Build history of the part. All positions in model axes, mm. A direction names the side the tool comes from. Give positions to 0.01 mm unless a question says otherwise; leave off trailing zeros. Order: outer loops, then holes, each group sorted by start corner. A loop starts at its lowest first (then second) coordinate and runs counter-clockwise, first axis right, second up. Notation, with made-up numbers: (31, 80) -> (44, 80) arc R16 ccw to (44, 98) -> close; hole circle Ø2 at (-24, 47). An arc over 180 degrees is marked (long way). Use a Markdown table: item, result. Add a question column.
Autodesk Inventor part; units mm, degrees
ref_plane "YZ Plane" through (0, 0, 0) normal (1, 0, 0) x (0, 1, 0)
ref_plane "XZ Plane" through (0, 0, 0) normal (0, 1, 0) x (-1, 0, 0)
ref_plane "XY Plane" through (0, 0, 0) normal (0, 0, 1) x (1, 0, 0)
sketch "Sketch12" plane through (0, 0, 0) normal (0, 0, 1) x (1, 0, 0)
  arc A0 (0, -5.7547) -> (0, 5.7547) centre (0, 0) ccw
  arc A1 (-12.7, 5.7547) -> (-12.7, -5.7547) centre (-12.7, 0) ccw
  line L0 (0, 5.7547) -> (-12.7, 5.7547)
  line L1 (0, -5.7547) -> (-12.7, -5.7547)
  dimension "d105" = 5.7547
  dimension "d106" = 12.7
extrude "Extrusion9" add sketch "Sketch12" along normal blind 1.5875
sketch "Sketch13" plane through (0, 0, 0) normal (0, 0, -1) x (-1, 0, 0)
  arc A0 (0, 5.7547) -> (0, -5.7547) centre (0, 0) ccw
  circle A1 centre (0, 0) radius 3.9688
  arc A2 (12.7, -5.7547) -> (12.7, 5.7547) centre (12.7, 0) ccw
  circle A3 centre (12.7, 0) radius 3.9688
  dimension "d109" = 7.9375
  dimension "d110" = 7.9375
extrude "Extrusion10" add sketch "Sketch13" along normal blind 12.7
sketch "Sketch14" plane through (0, 0, -12.7) normal (0, 0, -1) x (-1, 0, 0)
  circle A0 centre (0, 0) radius 3.9687
  circle A1 centre (0, 3.9687) radius 0.4536
  circle A2 centre (12.7, 0) radius 3.9687
  circle A3 centre (12.7, 3.9687) radius 0.4536
  circle A4 centre (-1.5188, 3.6666) radius 0.4536
  circle A5 centre (-2.8063, 2.8063) radius 0.4536
  circle A6 centre (-3.6666, 1.5188) radius 0.4536
  circle A7 centre (-3.9687, 0) radius 0.4536
  circle A8 centre (-3.6666, -1.5188) radius 0.4536
  circle A9 centre (-2.8063, -2.8063) radius 0.4536
  circle A10 centre (-1.5188, -3.6666) radius 0.4536
  circle A11 centre (0, -3.9687) radius 0.4536
  circle A12 centre (1.5188, -3.6666) radius 0.4536
  circle A13 centre (2.8063, -2.8063) radius 0.4536
  circle A14 centre (3.6666, -1.5188) radius 0.4536
  circle A15 centre (11.1812, 3.6666) radius 0.4536
  circle A16 centre (9.8937, 2.8063) radius 0.4536
  circle A17 centre (9.0334, 1.5188) radius 0.4536
  circle A18 centre (8.7313, 0) radius 0.4536
  circle A19 centre (9.0334, -1.5188) radius 0.4536
  circle A20 centre (9.8937, -2.8063) radius 0.4536
  circle A21 centre (11.1812, -3.6666) radius 0.4536
  circle A22 centre (12.7, -3.9688) radius 0.4536
  circle A23 centre (14.2188, -3.6666) radius 0.4536
  circle A24 centre (15.5063, -2.8063) radius 0.4536
  circle A25 centre (16.3666, -1.5188) radius 0.4536
  circle A26 centre (3.9687, 0) radius 0.4536
  circle A27 centre (3.6666, 1.5188) radius 0.4536
  circle A28 centre (2.8063, 2.8063) radius 0.4536
  circle A29 centre (1.5188, 3.6666) radius 0.4536
  circle A30 centre (16.6688, 0) radius 0.4536
  circle A31 centre (16.3666, 1.5188) radius 0.4536
  circle A32 centre (15.5063, 2.8063) radius 0.4536
  circle A33 centre (14.2188, 3.6666) radius 0.4536
  dimension "d113" = 0.9071
  dimension "d114" = 0.9071
  dimension "d117" = 360
  dimension "d121" = 360
sketch "Sketch15" plane through (0, 0, -12.7) normal (0, 0, -1) x (-1, 0, 0)
  circle A0 centre (0, 0) radius 0.9922
  arc A1 (12.7, -5.7547) -> (12.7, 5.7547) centre (12.7, 0) ccw
  circle A2 centre (12.7, 0) radius 0.9922
  dimension "d125" = 1.9844
  dimension "d126" = 1.9844
extrude "Extrusion12" cut sketch "Sketch15" against normal blind 4.7625
extrude "Extrusion14" cut sketch "Sketch14" against normal up to surface (12.7 mm away) contours A0 A26 | A0 A26 | A27 A0 | A0 A27 | A14 A0 | A0 A14 | A28 A0 | A0 A28 | A13 A0 | A0 A13 | A29 A0 | A0 A29 | A12 A0 | A0 A12 | A1 A0 | A0 A1 | A11 A0 | A0 A11 | A4 A0 | A0 A4 | A10 A0 | A0 A10 | A5 A0 | A0 A5 | A9 A0 | A0 A9 | A6 A0 | A0 A6 | A8 A0 | A0 A8 | A7 A0 | A0 A7 | A2 A30 | A2 A30 | A31 A2 | A2 A31 | A25 A2 | A2 A25 | A32 A2 | A2 A32 | A24 A2 | A2 A24 | A33 A2 | A2 A33 | A23 A2 | A2 A23 | A3 A2 | A2 A3 | A22 A2 | A2 A22 | A15 A2 | A2 A15 | A21 A2 | A2 A21 | A16 A2 | A2 A16 | A20 A2 | A2 A20 | A17 A2 | A2 A17 | A19 A2 | A2 A19 | A18 A2 | A2 A18
equation "\"d110\" = d109"
equation "\"d114\" = d113"
equation "\"d126\" = d125"
properties part number "arm-base"
(1) Pin check, flat tips, straight feed: pin 1 Ø1 at (x, z) = (-15.5, -5.5) entering from +Y; pin 2 Ø2.5 at (x, y) = (-12.7, 0) entering from -Z; pin 3 Ø2 at (y, z) = (-4, -1.5) entering from +X; pin 4 Ø1 at (x, z) = (-9, -3) entering from -Y. Stop position of each tip, or through.
(2) Band-saw the part on B-B on z = -11. State how many separate pieces and enclosed holes the cut face has, plus the area to 3 significant figures.
(3) Band-saw the part on A-A on y = 0. Give the cut face in (x, z), plus the area to 3 significant figures.
(4) Band-saw the part on C-C on x = -12. Give the cut face in (y, z).
(5) Band-saw the part on D-D on y = 2.75. Give the cut face in (x, z).
(6) Tool access for faces 1 (the face through (-6, 5.755, 1)), 2 (the face through (0.01, 3.515, -6.439)), 3 (the face through (-9.456, -1.354, -6.439)): list every direction of +Z, -Z, +X, -X, +Y, -Y with a clear straight run to the whole face (end or side of a thin tool).
(7) Mould opens along X. For faces 4 (the face through (3.25, 1.34, -6.44)), 5 (the face through (3.515, -0.01, -6.439)), 6 (the face through (-16.215, 0.01, -6.439)) say: released by +X, released by -X, zero draft, split by the parting line, or undercut.
(8) Wall check: probe 1 along Y at (x, z) = (0, -9.75); probe 2 along X at (y, z) = (0, -7.75); probe 3 along Y at (x, z) = (-16, -0.5). Give the ranges that are in metal, low to high.
Response:
| question | item | result |
|---|---|---|
| 1 | pin 1 | stops at y = 3.23 |
| 1 | pin 2 | stops at z = -12.7 |
| 1 | pin 3 | stops at x = 2.47 |
| 1 | pin 4 | stops at y = -2.35 |
| 2 | separate pieces | 2 |
| 2 | enclosed holes | 2 |
| 2 | area | 82.7 mm² |
| 3 | outline | (-18.45, 0) -> (-16.22, 0) -> (-16.22, -12.7) -> (-13.69, -12.7) -> (-13.69, -7.94) -> (-11.71, -7.94) -> (-11.71, -12.7) -> (-9.18, -12.7) -> (-9.18, 0) -> (-3.52, 0) -> (-3.52, -12.7) -> (-0.99, -12.7) -> (-0.99, -7.94) -> (0.99, -7.94) -> (0.99, -12.7) -> (3.52, -12.7) -> (3.52, 0) -> (5.75, 0) -> (5.75, 1.59) -> (-18.45, 1.59) -> close |
| 3 | area | 198 mm² |
| 4 | outline | (-5.75, 0) -> (-3.91, 0) -> (-3.91, -12.7) -> (-0.7, -12.7) -> (-0.7, -7.94) -> (0.7, -7.94) -> (0.7, -12.7) -> (3.91, -12.7) -> (3.91, 0) -> (5.75, 0) -> (5.75, 1.59) -> (-5.75, 1.59) -> close |
| 5 | outline | (-17.76, 0) -> (-15.06, 0) -> (-15.06, -12.7) -> (-10.34, -12.7) -> (-10.34, 0) -> (-2.36, 0) -> (-2.36, -12.7) -> (2.36, -12.7) -> (2.36, 0) -> (5.06, 0) -> (5.06, 1.59) -> (-17.76, 1.59) -> close |
| 6 | face 1 | +Z, -Z, +X, -X, +Y |
| 6 | face 2 | -Z, +Y |
| 6 | face 3 | -Z |
| 7 | face 4 | undercut |
| 7 | face 5 | released by +X |
| 7 | face 6 | released by -X |
| 8 | probe 1 | y = -3.52 to -0.99, 0.99 to 3.52 |
| 8 | probe 2 | x = -16.22 to -9.18, -3.52 to 3.52 |
| 8 | probe 3 | y = -2.2 to -1.79, -1.25 to 1.25, 1.79 to 2.2 |
